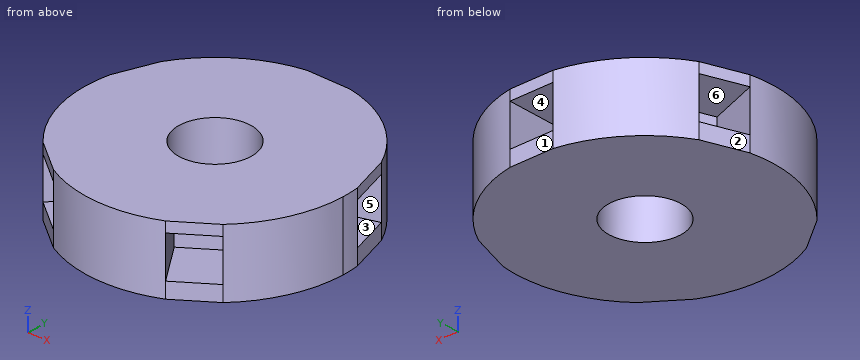
```python
from build123d import *

# Parameters (mm, degrees)
F0_R     = 3.5
F1_DEPTH = 6.5
F2_START = 1.5
F2_DEPTH = 4


with BuildPart() as f1:
    # F0 (on Top) → F1 (new body)
    with BuildSketch(Plane.XY):
        with BuildLine():
            Line((-9.1673866339, -8.4975892055), (-6.0491072211, -4.4337683552))
            ThreePointArc((-6.0491072211, -4.4337683552), (-7.2003739079, -2.0987176052), (-7.4840272858, 0.4892193627))
            Line((-7.4840272858, 0.4892193627), (-12.2974468195, 2.241160798))
            ThreePointArc((-12.2974468195, 2.241160798), (-12.0006231798, -3.4978626754), (-9.1673866339, -8.4975892055))
        make_face()
        with BuildLine():
            ThreePointArc((-6.0475616592, 4.4358762356), (-4.3018232726, 6.1436403322), (-2.0999722599, 7.2000080908))
            Line((-2.0999722599, 7.2000080908), (-2.0999722599, 12.3223421681))
            ThreePointArc((-2.0999722599, 12.3223421681), (-7.1697054544, 10.2394005536), (-10.8609811929, 6.1878176709))
            Line((-10.8609811929, 6.1878176709), (-6.0475616592, 4.4358762356))
        make_face()
        with BuildLine():
            ThreePointArc((2.0999722599, 7.2000080908), (4.4348223627, 6.048334532), (6.2352959244, 4.1678633297))
            Line((6.2352959244, 4.1678633297), (11.1205527613, 5.7081788938))
            ThreePointArc((11.1205527613, 5.7081788938), (7.3913706045, 10.0805575533), (2.0999722599, 12.3223421681))
            Line((2.0999722599, 12.3223421681), (2.0999722599, 7.2000080908))
        make_face()
        with BuildLine():
            ThreePointArc((7.4982435991, 0.1623050491), (7.4995608869, 0.0811572762), (7.5, 0))
            ThreePointArc((7.5, 0), (7.0754730103, -2.4875051115), (5.849951552, -4.6934067412))
            Line((5.849951552, -4.6934067412), (8.7880016779, -8.8893771722))
            ThreePointArc((8.7880016779, -8.8893771722), (11.5347306205, -4.8166367429), (12.5, 0))
            ThreePointArc((12.5, 0), (12.4708410993, 0.8533008116), (12.383500436, 1.7026206131))
            Line((12.383500436, 1.7026206131), (7.4982435991, 0.1623050491))
        make_face()
        with BuildLine():
            Line((5.3476085387, -11.2983663827), (2.4095584128, -7.1023959517))
            ThreePointArc((2.4095584128, -7.1023959517), (-0.1636116378, -7.4982152031), (-2.7170672074, -6.9905325828))
            Line((-2.7170672074, -6.9905325828), (-5.8353466201, -11.0543534331))
            ThreePointArc((-5.8353466201, -11.0543534331), (-0.2726860629, -12.4970253385), (5.3476085387, -11.2983663827))
        make_face()
        with BuildLine():
            ThreePointArc((-7.4840272858, 0.4892193627), (-7.0476946559, 2.5651510749), (-6.0475616592, 4.4358762356))
            Line((-6.0475616592, 4.4358762356), (-10.8609811929, 6.1878176709))
            Line((-10.8609811929, 6.1878176709), (-12.2974468195, 2.241160798))
            Line((-12.2974468195, 2.241160798), (-7.4840272858, 0.4892193627))
        make_face()
        with BuildLine():
            Line((8.7880016779, -8.8893771722), (5.849951552, -4.6934067412))
            ThreePointArc((5.849951552, -4.6934067412), (4.3018232726, -6.1436403322), (2.4095584128, -7.1023959517))
            Line((2.4095584128, -7.1023959517), (5.3476085387, -11.2983663827))
            Line((5.3476085387, -11.2983663827), (8.7880016779, -8.8893771722))
        make_face()
        with BuildLine():
            Line((-5.8353466201, -11.0543534331), (-2.7170672074, -6.9905325828))
            ThreePointArc((-2.7170672074, -6.9905325828), (-4.5657107176, -5.9501500522), (-6.0491072211, -4.4337683552))
            Line((-6.0491072211, -4.4337683552), (-9.1673866339, -8.4975892055))
            Line((-9.1673866339, -8.4975892055), (-5.8353466201, -11.0543534331))
        make_face()
        with BuildLine():
            Line((-7.4840272858, 0.4892193627), (-6.0475616592, 4.4358762356))
            ThreePointArc((-6.0475616592, 4.4358762356), (-7.0476946559, 2.5651510749), (-7.4840272858, 0.4892193627))
        make_face()
        with BuildLine():
            ThreePointArc((-2.0999722599, 7.2000080908), (0, 7.5), (2.0999722599, 7.2000080908))
            Line((2.0999722599, 7.2000080908), (2.0999722599, 12.3223421681))
            Line((2.0999722599, 12.3223421681), (-2.0999722599, 12.3223421681))
            Line((-2.0999722599, 12.3223421681), (-2.0999722599, 7.2000080908))
        make_face()
        with BuildLine():
            Line((-2.0999722599, 7.2000080908), (2.0999722599, 7.2000080908))
            ThreePointArc((2.0999722599, 7.2000080908), (0, 7.5), (-2.0999722599, 7.2000080908))
        make_face()
        with BuildLine():
            ThreePointArc((-6.0491072211, -4.4337683552), (-4.5657107176, -5.9501500522), (-2.7170672074, -6.9905325828))
            Line((-2.7170672074, -6.9905325828), (-6.0491072211, -4.4337683552))
        make_face()
        with BuildLine():
            ThreePointArc((5.849951552, -4.6934067412), (7.0754730103, -2.4875051115), (7.5, 0))
            ThreePointArc((7.5, 0), (7.4995608869, 0.0811572762), (7.4982435991, 0.1623050491))
            Line((7.4982435991, 0.1623050491), (6.2352959244, 4.1678633297))
            ThreePointArc((6.2352959244, 4.1678633297), (4.4348223627, 6.048334532), (2.0999722599, 7.2000080908))
            Line((2.0999722599, 7.2000080908), (-2.0999722599, 7.2000080908))
            ThreePointArc((-2.0999722599, 7.2000080908), (-4.3018232726, 6.1436403322), (-6.0475616592, 4.4358762356))
            Line((-6.0475616592, 4.4358762356), (-7.4840272858, 0.4892193627))
            ThreePointArc((-7.4840272858, 0.4892193627), (-7.2003739079, -2.0987176052), (-6.0491072211, -4.4337683552))
            Line((-6.0491072211, -4.4337683552), (-2.7170672074, -6.9905325828))
            ThreePointArc((-2.7170672074, -6.9905325828), (-0.1636116378, -7.4982152031), (2.4095584128, -7.1023959517))
            Line((2.4095584128, -7.1023959517), (5.849951552, -4.6934067412))
        make_face()
        Circle(F0_R, mode=Mode.SUBTRACT)
        with BuildLine():
            ThreePointArc((2.4095584128, -7.1023959517), (4.3018232726, -6.1436403322), (5.849951552, -4.6934067412))
            Line((5.849951552, -4.6934067412), (2.4095584128, -7.1023959517))
        make_face()
        with BuildLine():
            Line((6.2352959244, 4.1678633297), (7.4982435991, 0.1623050491))
            ThreePointArc((7.4982435991, 0.1623050491), (7.1528771306, 2.2552934963), (6.2352959244, 4.1678633297))
        make_face()
        with BuildLine():
            ThreePointArc((6.2352959244, 4.1678633297), (7.1528771306, 2.2552934963), (7.4982435991, 0.1623050491))
            Line((7.4982435991, 0.1623050491), (12.383500436, 1.7026206131))
            Line((12.383500436, 1.7026206131), (11.1205527613, 5.7081788938))
            Line((11.1205527613, 5.7081788938), (6.2352959244, 4.1678633297))
        make_face()
    extrude(amount=F1_DEPTH)

    # F0 (on Top) → F2 (cut)
    with BuildSketch(Plane.XY.offset(F2_START)):
        with BuildLine():
            Line((-5.8353466201, -11.0543534331), (-2.7170672074, -6.9905325828))
            ThreePointArc((-2.7170672074, -6.9905325828), (-4.5657107176, -5.9501500522), (-6.0491072211, -4.4337683552))
            Line((-6.0491072211, -4.4337683552), (-9.1673866339, -8.4975892055))
            Line((-9.1673866339, -8.4975892055), (-5.8353466201, -11.0543534331))
        make_face()
        with BuildLine():
            ThreePointArc((-6.0491072211, -4.4337683552), (-4.5657107176, -5.9501500522), (-2.7170672074, -6.9905325828))
            Line((-2.7170672074, -6.9905325828), (-6.0491072211, -4.4337683552))
        make_face()
        with BuildLine():
            ThreePointArc((-7.4840272858, 0.4892193627), (-7.0476946559, 2.5651510749), (-6.0475616592, 4.4358762356))
            Line((-6.0475616592, 4.4358762356), (-10.8609811929, 6.1878176709))
            Line((-10.8609811929, 6.1878176709), (-12.2974468195, 2.241160798))
            Line((-12.2974468195, 2.241160798), (-7.4840272858, 0.4892193627))
        make_face()
        with BuildLine():
            Line((-7.4840272858, 0.4892193627), (-6.0475616592, 4.4358762356))
            ThreePointArc((-6.0475616592, 4.4358762356), (-7.0476946559, 2.5651510749), (-7.4840272858, 0.4892193627))
        make_face()
        with BuildLine():
            ThreePointArc((-2.0999722599, 7.2000080908), (0, 7.5), (2.0999722599, 7.2000080908))
            Line((2.0999722599, 7.2000080908), (2.0999722599, 12.3223421681))
            Line((2.0999722599, 12.3223421681), (-2.0999722599, 12.3223421681))
            Line((-2.0999722599, 12.3223421681), (-2.0999722599, 7.2000080908))
        make_face()
        with BuildLine():
            Line((-2.0999722599, 7.2000080908), (2.0999722599, 7.2000080908))
            ThreePointArc((2.0999722599, 7.2000080908), (0, 7.5), (-2.0999722599, 7.2000080908))
        make_face()
        with BuildLine():
            ThreePointArc((6.2352959244, 4.1678633297), (7.1528771306, 2.2552934963), (7.4982435991, 0.1623050491))
            Line((7.4982435991, 0.1623050491), (12.383500436, 1.7026206131))
            Line((12.383500436, 1.7026206131), (11.1205527613, 5.7081788938))
            Line((11.1205527613, 5.7081788938), (6.2352959244, 4.1678633297))
        make_face()
        with BuildLine():
            Line((6.2352959244, 4.1678633297), (7.4982435991, 0.1623050491))
            ThreePointArc((7.4982435991, 0.1623050491), (7.1528771306, 2.2552934963), (6.2352959244, 4.1678633297))
        make_face()
        with BuildLine():
            Line((8.7880016779, -8.8893771722), (5.849951552, -4.6934067412))
            ThreePointArc((5.849951552, -4.6934067412), (4.3018232726, -6.1436403322), (2.4095584128, -7.1023959517))
            Line((2.4095584128, -7.1023959517), (5.3476085387, -11.2983663827))
            Line((5.3476085387, -11.2983663827), (8.7880016779, -8.8893771722))
        make_face()
        with BuildLine():
            ThreePointArc((2.4095584128, -7.1023959517), (4.3018232726, -6.1436403322), (5.849951552, -4.6934067412))
            Line((5.849951552, -4.6934067412), (2.4095584128, -7.1023959517))
        make_face()
    extrude(amount=F2_DEPTH, mode=Mode.SUBTRACT)


solid = f1.part
```
For this review, take the finished solid that the model builds, in its own axes (mm). Face numbers are marked on the shaded views. A direction names the side the tool comes from. Coordinates: 2 decimals unless noted, no trailing zeros. Order: outer loops, then holes, each group sorted by start corner. A loop starts at its lowest first (then second) coordinate and runs counter-clockwise, first axis right, second up. Notation, with made-up numbers: (67.25, 44) -> (112.25, 44) arc R20 cw to (112.25, 82) -> close; hole circle Ø11 at (-36.75, 71.25). An arc over 180 degrees is marked (long way). Use CSV: the item, a comma, the result in double quotes. Start each with the question number.
Item 1: For the marked faces 4, 5 and 6, list the 3-axis set-ups (+Z, -Z, +X, -X, +Y, -Y) from which the entire face can be reached by the end or side of a thin tool; tool diameter is ignored.
Item 2: We need section A-A, the plane z = 6. Give the boundary of the cut face in (x, y), then the cut area to 3 significant figures.
Item 3: We need section B-B, the plane x = 0. Give the boundary of the cut face in (y, z), then the cut area to 3 significant figures.
Item 4: We need section D-D, the plane y = 9. Give the boundary of the cut face in (x, z).
Item 5: We need section C-C, the plane x = -5.25. Give the boundary of the cut face in (y, z), then the cut area to 3 significant figures.
Item 6: Insertion check: pin 1 (2 mm diameter, centred on x = 0, z = 4, fed in from +Y); pin 2 (3 mm diameter, centred on y = 10, z = 2.5, fed in from -X). Each pin has a flat end and moves straight along its axis. Give the tip position at first contact, or say it passes through.
Item 7: Draft analysis for pull direction X (two halves, no side actions). For the marked faces 1, 2 and 3, state which applies: pulls with the +X half, pulls with the -X half, needs draft (parallel to the pull), parting line crosses it, or undercut.
Item 8: Wall thickness on probe 1 along Z at (x, y) = (-8.5, 2.5); probe 2 along Y at (x, z) = (0, 1.75); probe 3 along X at (y, z) = (8, 3.5): over which ranges is each line inside the solid? List them lowest first.
Derived:
1,face 4,"+Y"
1,face 5,"+X"
1,face 6,"none"
2,outline,"(-12.3, 2.24) arc R12.5 ccw to (-9.17, -8.5) -> (-5.84, -11.05) arc R12.5 ccw to (5.35, -11.3) -> (8.79, -8.89) arc R12.5 ccw to (12.38, 1.7) -> (11.12, 5.71) arc R12.5 ccw to (2.1, 12.32) -> (-2.1, 12.32) arc R12.5 ccw to (-10.86, 6.19) -> close; hole circle Ø7 at (0, 0)"
2,area,"450 mm^2"
3,outline,"(-12.5, 0) -> (-3.5, 0) -> (-3.5, 6.5) -> (-12.5, 6.5) -> close; (3.5, 0) -> (12.32, 0) -> (12.32, 1.5) -> (7.2, 1.5) -> (7.2, 5.5) -> (12.32, 5.5) -> (12.32, 6.5) -> (3.5, 6.5) -> close"
3,area,"95.4 mm^2"
4,outline,"(-8.67, 0) -> (8.67, 0) -> (8.67, 6.5) -> (-8.67, 6.5) -> close; hole (-2.1, 1.5) -> (2.1, 1.5) -> (2.1, 5.5) -> (-2.1, 5.5) -> close"
5,outline,"(-11.34, 0) -> (11.34, 0) -> (11.34, 6.5) -> (-11.34, 6.5) -> close; hole (-10.29, 1.5) -> (-5.05, 1.5) -> (-5.05, 5.5) -> (-10.29, 5.5) -> close"
5,area,"126 mm^2"
6,pin 1,"stops at y = 7.2"
6,pin 2,"stops at x = -9.17"
7,face 1,"needs draft"
7,face 2,"pulls with the -X half"
7,face 3,"undercut"
8,probe 1,"z = 0 to 1.5, 5.5 to 6.5"
8,probe 2,"y = -12.5 to -3.5, 3.5 to 7.2"
8,probe 3,"x = -9.6 to -2.1, 2.1 to 9.6"
